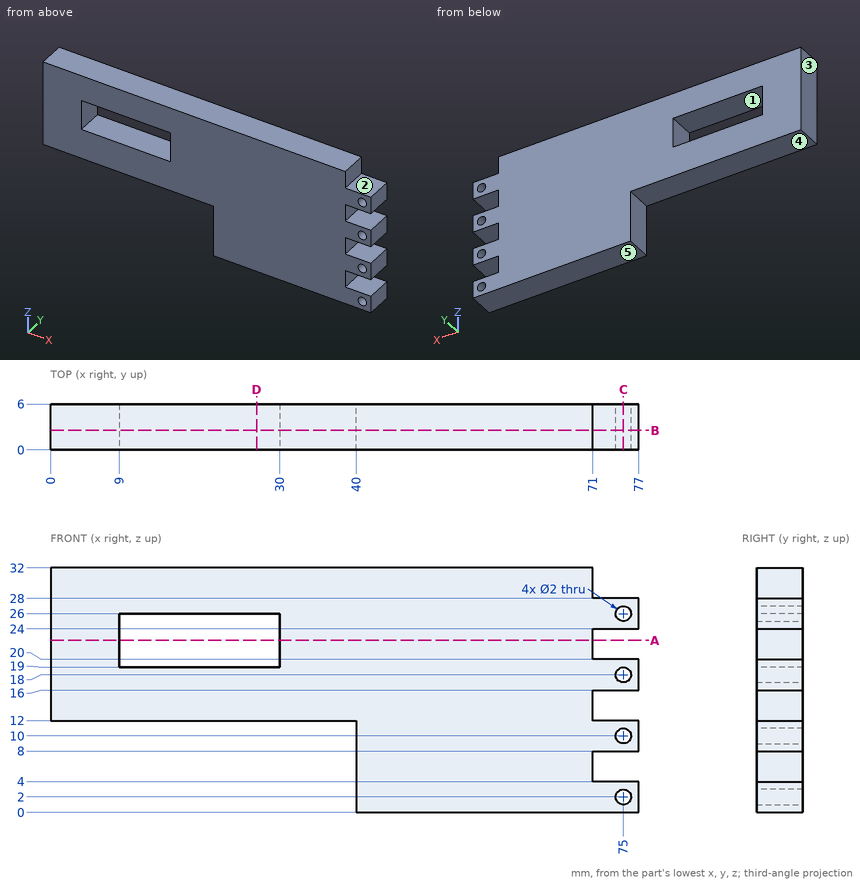
Geometry: see drawing. Coordinates: mm, zero at the bounding-box minimum. A direction names the side the tool comes from. Coordinates: 2 decimals unless noted, no trailing zeros. Loops run counter-clockwise (first coordinate to the right, second up) from the corner with the lowest first, then second, coordinate; pieces in that order, holes last. Notation, with made-up numbers: (22, -25.75) - (74, -25.75) arc R10 cw to (74, -18.75) - close; hole circle Ø2 at (-8.5, 40.25). An arc over 180 degrees is marked (long way). Return JSON: item names as keys, results as strings.
Q1. Access query for the marked faces 1, 2, 3, 4 and 5. Directions: +Z, -Z, +X, -X, +Y, -Y. A direction counts if a zero-diameter tool reaches every point of the face in a straight line with its end or side. Return the directions, or none.
Results:
{"face 1": "+Y, -Y", "face 2": "+Z, +X, +Y, -Y", "face 3": "+Z, -Z, -X, +Y, -Y", "face 4": "-Z, -X, +Y, -Y", "face 5": "-Z, +X, -X, +Y, -Y"}
Q2. Section A-A, the plane z = 22.5. Return loops of the section in (x, y), plus the area to 3 significant figures.
Results:
{"outline": "(0, 0) - (9, 0) - (9, 6) - (0, 6) - close; (30, 0) - (71, 0) - (71, 6) - (30, 6) - close", "area": "300 mm2"}
Q3. Material intervals for line 1 along X through (y, z) = (1.7, 18); line 2 along Z through (x, y) = (28, 0.5); line 3 along X through (y, z) = (4.65, 10), sorted ascending.
Results:
{"line 1": "0 to 74, 76 to 77", "line 2": "12 to 19, 26 to 32", "line 3": "40 to 74, 76 to 77"}
Q4. Contact query for flat-ended pins moving along their axis: P1, Ø2, axis at x = 28.5, y = 3, coming from the -Z side; P2, Ø3, axis at y = 1.5, z = 7, coming from the -X side; P3, Ø1.8, axis at x = 73, y = 3, coming from the +Z side. Output: stop coordinate, or through.
Results:
{"P1": "z = 12", "P2": "x = 40", "P3": "z = 28"}
Q5. Section C-C, the plane x = 75. Give the number of separate pieces and of enclosed holes in the cut face, plus the area to 3 significant figures.
Results:
{"separate pieces": "8", "enclosed holes": "0", "area": "48.0 mm2"}
Q6. Section B-B, the plane y = 2.55. Return loops of the section in (x, z).
Results:
{"outline": "(0, 12) - (40, 12) - (40, 0) - (77, 0) - (77, 4) - (71, 4) - (71, 8) - (77, 8) - (77, 12) - (71, 12) - (71, 16) - (77, 16) - (77, 20) - (71, 20) - (71, 24) - (77, 24) - (77, 28) - (71, 28) - (71, 32) - (0, 32) - close; hole (9, 19) - (30, 19) - (30, 26) - (9, 26) - close; hole circle Ø2 at (75, 2); hole circle Ø2 at (75, 10); hole circle Ø2 at (75, 18); hole circle Ø2 at (75, 26)"}
Q7. Section D-D, the plane x = 27. Return loops of the section in (y, z).
Results:
{"outline": "(0, 12) - (6, 12) - (6, 19) - (0, 19) - close; (0, 26) - (6, 26) - (6, 32) - (0, 32) - close"}
